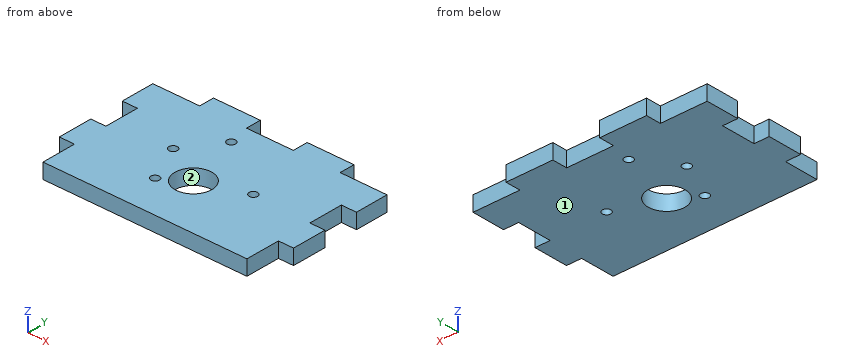
```python
from build123d import *

# Parameters (mm, degrees)
SKETCH1_W                = 82.55
SKETCH1_H                = 53.594
BOSS_EXTRUDE1_DEPTH      = 5.334
CUT_EXTRUDE1_START       = -88.085249325
CUT_EXTRUDE1_OUTLINE_W   = 5.334
CUT_EXTRUDE1_OUTLINE_H   = 5.334
CUT_EXTRUDE1_DEPTH       = 16.51
CUT_EXTRUDE1_START_2     = -55.065249325
CUT_EXTRUDE1_2_OUTLINE_W = 5.334
CUT_EXTRUDE1_2_OUTLINE_H = 5.334
CUT_EXTRUDE1_2_DEPTH     = 16.51
CUT_EXTRUDE1_START_3     = -22.045249325
CUT_EXTRUDE1_3_OUTLINE_W = 5.334
CUT_EXTRUDE1_3_OUTLINE_H = 5.334
CUT_EXTRUDE1_3_DEPTH     = 16.51
SKETCH3_W                = 5.334
SKETCH3_H                = 12.154056038
CUT_EXTRUDE2_DEPTH       = 97.676684204
SKETCH5_R                = 1.5
SKETCH5_R_2              = 6.5
CUT_EXTRUDE4_DEPTH       = 97.676684204


# Read off the part's stored shape, not the designer's step: Cut-Extrude1
with BuildPart() as part:
    # Sketch1 → Boss-Extrude1 (new body)
    with BuildSketch(Plane.XY):
        with Locations((-46.810249325, -12.686142782)):
            Rectangle(SKETCH1_W, SKETCH1_H)
    extrude(amount=BOSS_EXTRUDE1_DEPTH)

    # Cut-Extrude1 outline → Cut-Extrude1 (cut)
    with BuildSketch(Plane.YZ.offset(CUT_EXTRUDE1_START)):
        with Locations((11.443857218, 2.667)):
            Rectangle(CUT_EXTRUDE1_OUTLINE_W, CUT_EXTRUDE1_OUTLINE_H)
    extrude(amount=CUT_EXTRUDE1_DEPTH, mode=Mode.SUBTRACT)

    # Cut-Extrude1 2 outline → Cut-Extrude1 2 (cut)
    with BuildSketch(Plane.YZ.offset(CUT_EXTRUDE1_START_2)):
        with Locations((11.443857218, 2.667)):
            Rectangle(CUT_EXTRUDE1_2_OUTLINE_W, CUT_EXTRUDE1_2_OUTLINE_H)
    extrude(amount=CUT_EXTRUDE1_2_DEPTH, mode=Mode.SUBTRACT)

    # Cut-Extrude1 3 outline → Cut-Extrude1 3 (cut)
    with BuildSketch(Plane.YZ.offset(CUT_EXTRUDE1_START_3)):
        with Locations((11.443857218, 2.667)):
            Rectangle(CUT_EXTRUDE1_3_OUTLINE_W, CUT_EXTRUDE1_3_OUTLINE_H)
    extrude(amount=CUT_EXTRUDE1_3_DEPTH, mode=Mode.SUBTRACT)

    # Sketch3 → Cut-Extrude2 (cut, through all)
    with BuildSketch(Plane.XY.offset(5.334)):
        with Locations((-85.418249325, -33.406114763)):
            Rectangle(SKETCH3_W, SKETCH3_H)
        with Locations((-85.418249325, -9.098002686)):
            Rectangle(SKETCH3_W, SKETCH3_H)
        with Locations((-8.202249325, -33.406114763)):
            Rectangle(SKETCH3_W, SKETCH3_H)
        with Locations((-8.202249325, -9.098002686)):
            Rectangle(SKETCH3_W, SKETCH3_H)
    extrude(amount=-CUT_EXTRUDE2_DEPTH, mode=Mode.SUBTRACT)

    # Sketch5 → Cut-Extrude4 (cut, through all)
    with BuildSketch(Plane.XY.offset(5.334)):
        with Locations((-62.244676311, -11.668301366)):
            Circle(SKETCH5_R)
        with Locations((-55.760892065, -25.747027937)):
            Circle(SKETCH5_R)
        with Locations((-53.29403357, 0.986183789)):
            Circle(SKETCH5_R)
        with Locations((-31.375822338, -14.516784198)):
            Circle(SKETCH5_R)
        with Locations((-47.453455125, -20.062929163)):
            Circle(SKETCH5_R_2)
    extrude(amount=-CUT_EXTRUDE4_DEPTH, mode=Mode.SUBTRACT)


solid = part.part
```
For this review, take the finished solid that the model builds, in its own axes (mm). Face numbers are marked on the shaded views. Round coordinates to 2 decimals unless told otherwise and drop trailing zeros. Loops run counter-clockwise (first coordinate to the right, second up) from the corner with the lowest first, then second, coordinate; pieces in that order, holes last.
(1) We need section A-A (x = -47). Give the boundary of the cut face in (y, z), plus the area to 3 significant figures.
Returned:
outline: (-39.48, 0) - (-26.55, 0) - (-26.55, 5.33) - (-39.48, 5.33) - close; (-13.58, 0) - (8.78, 0) - (8.78, 5.33) - (-13.58, 5.33) - close
area: 188 mm2
(2) Mouldability with a two-part tool opening along X and no side actions: class the marked faces 1 and 2 as released by +X, released by -X, zero draft, split by the parting line, or undercut.
Returned:
face 1: zero draft
face 2: undercut
(3) Clearance check with flat-ended pins moving along their axes: P1, Ø1.6, axis at x = -9, z = 1.5, coming from the +Y side; P2, Ø1.5, axis at y = -7.5, z = 4, coming from the -X side; P3, Ø2.5, axis at y = 10.5, z = 1.5, coming from the -X side. State where each tip first meets the part, or that it passes through.
Returned:
P1: stops at y = 8.78
P2: stops at x = -82.75
P3: stops at x = -71.58
(4) We need section C-C (y = -29.5). Give the boundary of the cut face in (x, z).
Returned:
outline: (-82.75, 0) - (-10.87, 0) - (-10.87, 5.33) - (-82.75, 5.33) - close
(5) Wall thickness on line 1 along X through (y, z) = (-31, 4.8); line 2 along Y through (x, z) = (-31.5, 4.7); line 3 along Y through (x, z) = (-14, 4.1): over which ranges is each line inside the solid? List them lowest first.
Returned:
line 1: x = -82.75 to -10.87
line 2: y = -39.48 to -16.01, -13.02 to 14.11
line 3: y = -39.48 to 8.78
(6) We need section B-B (z = 3.5). State how many separate pieces and enclosed holes the cut face has, plus the area to 3 significant figures.
Returned:
separate pieces: 1
enclosed holes: 5
area: 3,740 mm2
